Design review of the part built by this model. Coordinates are the model's own, in mm. A direction names the side the tool comes from. Give positions to 0.01 mm unless a question says otherwise; leave off trailing zeros. Loops run counter-clockwise (first coordinate to the right, second up) from the corner with the lowest first, then second, coordinate; pieces in that order, holes last. Notation, with made-up numbers: (-16, 70) - (1, 70) arc R30 ccw to (1, 105) - close; hole circle Ø5 at (55, 76). An arc over 180 degrees is marked (long way). Put each result on its own line as item: value. Start each with the question number.
Autodesk Inventor part; units mm, degrees
ref_plane "YZ Plane" through (0, 0, 0) normal (1, 0, 0) x (0, 1, 0)
ref_plane "XZ Plane" through (0, 0, 0) normal (0, 1, 0) x (-1, 0, 0)
ref_plane "XY Plane" through (0, 0, 0) normal (0, 0, 1) x (1, 0, 0)
sketch "Sketch1" plane through (0, 0, 0) normal (0, 0, 1) x (1, 0, 0)
  line L0 (0, 0) -> (-26, 0)
  line L1 (0, 0) -> (0, 36.5)
  line L2 (0, 36.5) -> (-26, 36.5)
  line L3 (-26, 36.5) -> (-26, 0)
  dimension "d0" = 26
  dimension "d1" = 36.5
sketch "Sketch2" plane through (0, 0, 0) normal (0, 0, 1) x (1, 0, 0)
  line L0 (-13, 0) -> (-13, 6.25)
  circle A0 centre (-21, 30.25) radius 1.7
  circle A1 centre (-21, 6.25) radius 1.7
  circle A2 centre (-5, 30.25) radius 1.7
  circle A3 centre (-5, 6.25) radius 1.7
  line L1 (-13, 6.25) -> (-5, 6.25)
  line L2 (-13, 6.25) -> (-21, 6.25)
  line L3 (-21, 30.25) -> (-5, 30.25)
  line L4 (-5, 30.25) -> (-5, 6.25)
  line L5 (-21, 18.25) -> (-13, 18.25)
  line L6 (-13, 18.25) -> (-13, 6.25)
  line L7 (-21, 6.25) -> (-21, 18.25)
  line L8 (-21, 18.25) -> (-21, 30.25)
  line L9 (0, 0) -> (-13, 0)
  line L10 (-18.075, 4.5613) -> (-21, 2.8725)
  line L11 (-21, 2.8725) -> (-23.925, 4.5613)
  line L12 (-23.925, 4.5613) -> (-23.925, 7.9387)
  line L13 (-23.925, 7.9387) -> (-21, 9.6275)
  line L14 (-21, 9.6275) -> (-18.075, 7.9387)
  line L15 (-18.075, 7.9387) -> (-18.075, 4.5613)
  line L16 (-7.925, 7.9387) -> (-5, 9.6275)
  line L17 (-5, 9.6275) -> (-2.075, 7.9387)
  line L18 (-2.075, 7.9387) -> (-2.075, 4.5613)
  line L19 (-2.075, 4.5613) -> (-5, 2.8725)
  line L20 (-5, 2.8725) -> (-7.925, 4.5613)
  line L21 (-7.925, 4.5613) -> (-7.925, 7.9387)
  line L22 (-7.925, 31.9387) -> (-5, 33.6275)
  line L23 (-5, 33.6275) -> (-2.075, 31.9387)
  line L24 (-2.075, 31.9387) -> (-2.075, 28.5613)
  line L25 (-2.075, 28.5613) -> (-5, 26.8725)
  line L26 (-5, 26.8725) -> (-7.925, 28.5613)
  line L27 (-7.925, 28.5613) -> (-7.925, 31.9387)
  line L28 (-18.075, 28.5613) -> (-21, 26.8725)
  line L29 (-21, 26.8725) -> (-23.925, 28.5613)
  line L30 (-23.925, 28.5613) -> (-23.925, 31.9387)
  line L31 (-23.925, 31.9387) -> (-21, 33.6275)
  line L32 (-21, 33.6275) -> (-18.075, 31.9387)
  line L33 (-18.075, 31.9387) -> (-18.075, 28.5613)
  point P0 (8.2274, 51.4671)
  point P1 (-18.075, 6.25)
  point P2 (-7.925, 6.25)
  point P3 (-7.925, 30.25)
  point P4 (-18.075, 30.25)
  dimension "d2" = 3.4
  dimension "d3" = 3.4
  dimension "d4" = 3.4
  dimension "d5" = 3.4
  dimension "d7" = 8
  dimension "d8" = 8
  dimension "d9" = 12
  dimension "d10" = 12
  dimension "d12" = 18.25
  dimension "d13" = 13
  dimension "d34" = 5.85
  dimension "d35" = 5.85
  dimension "d36" = 5.85
  dimension "d37" = 5.85
extrude "Extrusion1" add sketch "Sketch1" along normal blind 5
hole "Hole1" at (8.2274, 51.4671, 0) at (-5, 30.25, 0) at (-21, 30.25, 0) at (-21, 6.25, 0) at (-5, 6.25, 0) direction (0, 0, 1) diameter 3.4 end through all
chamfer "Chamfer1" distance 3 angle 45 4 edges at (0, 0, 2.5) (-26, 0, 2.5) (-26, 36.5, 2.5) (0, 36.5, 2.5)
extrude "Extrusion3" cut sketch "Sketch2" along normal blind 2 contours L3 L33 L28 L8 A0 | A0 L8 L29 L30 L31 L32 L33 L3 | L27 L22 L23 L24 L25 L4 A2 L3 | L3 A2 L4 L26 L27 | L14 L15 L2 A1 L7 | L7 A1 L2 L15 L10 L11 L12 L13 | L17 L18 L19 L20 L21 L1 A3 L4 | L4 A3 L1 L21 L16
chamfer "Chamfer2" distance 1 angle 45 8 edges at (-1.5, 1.5, 0) (-13, 0, 0) (-24.5, 1.5, 0) (-26, 18.25, 0) (-13, 36.5, 0) (-1.5, 35, 0) (-24.5, 35, 0) (0, 18.25, 0)
equation "\"d3\" = d2"
equation "\"d4\" = d2"
equation "\"d5\" = d2"
equation "\"d8\" = d7"
equation "\"d9\" = d10"
equation "\"d13\" = 0.5 * d0"
equation "\"d35\" = d34"
equation "\"d36\" = d34"
equation "\"d37\" = d34"
equation "\"d16\" = d2"
properties part number "camera_adapter"
Item 1: Consider section A-A (y = 30.25). State the section outline as (x, z) points (3 decimals).
Item 2: Mouldability with a two-part tool opening along X and no side actions: class faces 1 (the flat face through (-1.828, 34.63, 0.507)), 2 (the flat face through (-19.7, 4.8, 2)), 3 (the flat face through (-24.13, 1.828, 0.507)) as pulls with the +X half, pulls with the -X half, needs draft (parallel to the pull), parting line crosses it, or undercut.
Item 3: Machinability: for faces 4 (the flat face through (-18.075, 6, 1)), 5 (the flat face through (-24.5, 35, 3)), which of the approach directions +Z, -Z, +X, -X, +Y, -Y give a long, thin tool a straight path to every point of the face, cutting with its end or side? Answer none if there is none.
Item 4: Consider section B-B (z = 3.2). State the section outline as (x, y) points, plus the area to 3 significant figures.
Item 5: For P1, Ø3, axis at x = -21.5, y = 6, coming from the -Z side; P2, Ø2, axis at x = -21, y = 6.25, coming from the +Z side, all flat-tipped, find the tip position at first contact; note any pin that passes through.
Item 6: For L1, parallel to Y at x = -5, z = 2.6; L2, parallel to X at y = 6.25, z = 2.8; L3, parallel to X at y = 29.5, z = 2.3, list the stretches that pass through material, from the lowest coordinate up. Write a range as from..to.
Item 7: Consider section C-C (y = 5). State the section outline as (x, z) points (3 decimals), plus the area to 3 significant figures.
Geometry says:
1. outline: (-26, 1) - (-25, 0) - (-23.925, 0) - (-23.925, 2) - (-22.7, 2) - (-22.7, 5) - (-26, 5) - close; (-19.3, 2) - (-18.075, 2) - (-18.075, 0) - (-7.925, 0) - (-7.925, 2) - (-6.7, 2) - (-6.7, 5) - (-19.3, 5) - close; (-3.3, 2) - (-2.075, 2) - (-2.075, 0) - (-1, 0) - (0, 1) - (0, 5) - (-3.3, 5) - close
2. face 1: pulls with the +X half
2. face 2: undercut
2. face 3: pulls with the -X half
3. face 4: -Z
3. face 5: +Z, -Z, -X, +Y
4. outline: (-26, 3) - (-23, 0) - (-3, 0) - (0, 3) - (0, 33.5) - (-3, 36.5) - (-23, 36.5) - (-26, 33.5) - close; hole circle Ø3.4 at (-21, 6.25); hole circle Ø3.4 at (-21, 30.25); hole circle Ø3.4 at (-5, 6.25); hole circle Ø3.4 at (-5, 30.25)
4. area: 895 mm2
5. P1: stops at z = 2
5. P2: passes through
6. L1: y = 0..4.55, 7.95..28.55, 31.95..36.5
6. L2: x = -26..-22.7, -19.3..-6.7, -3.3..0
6. L3: x = -26..-22.53, -19.47..-6.53, -3.47..0
7. outline: (-26, 1) - (-25, 0) - (-23.925, 0) - (-23.925, 2) - (-22.152, 2) - (-22.152, 5) - (-26, 5) - close; (-19.848, 2) - (-18.075, 2) - (-18.075, 0) - (-7.925, 0) - (-7.925, 2) - (-6.152, 2) - (-6.152, 5) - (-19.848, 5) - close; (-3.848, 2) - (-2.075, 2) - (-2.075, 0) - (-1, 0) - (0, 1) - (0, 5) - (-3.848, 5) - close
7. area: 91.8 mm2
